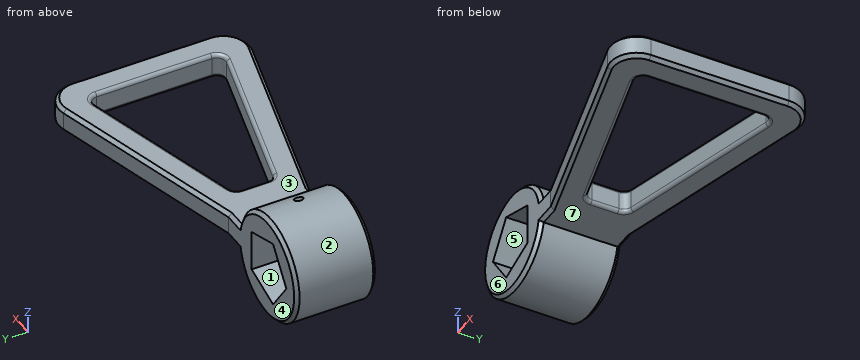
```python
from build123d import *

# Parameters (mm, degrees)
BOSS_EXTRUDE2_DEPTH     = 7
SKETCH2_R               = 30
BOSS_EXTRUDE4_DEPTH     = 23
CUT_EXTRUDE1_DEPTH      = 46
CUT_EXTRUDE2_REACH      = 185.241
CUT_EXTRUDE2_END_RADIUS = 30
SKETCH4_R               = 2.5
FILLET1_R               = 5
CHAMFER1_SIZE           = 2
FILLET2_R               = 2


with BuildPart() as part:
    # Sketch1 → Boss-Extrude2 (new, symmetric)
    with BuildSketch(Plane.XY):
        with BuildLine():
            Line((174, -39.356811193), (174, 39.356811193))
            ThreePointArc((174, 39.356811193), (168.131421435, 51.257111298), (155.117714323, 53.845698587))
            Line((155.117714323, 53.845698587), (40, 23))
            Line((40, 23), (30, 23))
            Line((30, 23), (0, 23))
            Line((0, 23), (0, -23))
            Line((0, -23), (30, -23))
            Line((30, -23), (40, -23))
            Line((40, -23), (155.117714323, -53.845698587))
            ThreePointArc((155.117714323, -53.845698587), (168.131421435, -51.257111298), (174, -39.356811193))
        make_face()
        Polygon((159, -39.356811193), (159, 39.356811193), (55, 11.49009518), (55, -11.49009518), align=None, mode=Mode.SUBTRACT)
    extrude(amount=BOSS_EXTRUDE2_DEPTH, both=True)

    # Sketch2 → Boss-Extrude4 (add, symmetric)
    with BuildSketch(Plane(origin=(0, 0, 0), x_dir=(1, 0, 0), z_dir=(0, 1, 0))):
        Circle(SKETCH2_R)
    extrude(amount=BOSS_EXTRUDE4_DEPTH, both=True)

    # Sketch3 → Cut-Extrude1 (cut)
    with BuildSketch(Plane(origin=(0, 23, 0), x_dir=(1, 0, 0), z_dir=(0, 1, 0))):
        Polygon((16.099689438, 11.697109064), (-6.149534157, 18.926320036), (-19.900310562, 0), (-6.149534157, -18.926320036), (16.099689438, -11.697109064), align=None)
    extrude(amount=-CUT_EXTRUDE1_DEPTH, mode=Mode.SUBTRACT)

    # Cut-Extrude2: up to this cylinder (the profile starts inside it)
    cut_extrude2_end = Plane(origin=(0, 0, 0), z_dir=(0, -1, 0)) * Cylinder(CUT_EXTRUDE2_END_RADIUS, 431.482, mode=Mode.PRIVATE)
    # Sketch4 → Cut-Extrude2 (cut, up to the surface)
    with BuildSketch(Plane(origin=(4.975077641, 0, 15.31171455), x_dir=(-0.9510565162951536, 0, 0.30901699437494745), z_dir=(-0.3090169943749474, 0, -0.9510565162951535)), mode=Mode.PRIVATE) as cut_extrude2_sk1:
        Circle(SKETCH4_R)
    cut_extrude2_tool1 = extrude(cut_extrude2_sk1.sketch, amount=-CUT_EXTRUDE2_REACH, mode=Mode.PRIVATE) & cut_extrude2_end
    add(cut_extrude2_tool1.solids().sort_by_distance((4.975078, 0, 15.311715))[0], mode=Mode.SUBTRACT)

    # Fillet1
    fillet1_edges = [part.edges().sort_by_distance(p)[0] for p in [
        (55, -11.49009518, 0),
        (159, -39.356811193, 0),
        (159, 39.356811193, 0),
        (55, 11.49009518, 0),
    ]]
    fillet(fillet1_edges, radius=FILLET1_R)

    # Chamfer1
    chamfer1_edges = [part.edges().sort_by_distance(p)[0] for p in [
        (34.585952146, 23, 7),
        (97.558857162, -38.422849294, -7),
        (34.585952146, 23, -7),
        (97.558857162, 38.422849294, -7),
        (168.131421435, 51.257111298, -7),
        (97.558857162, -38.422849294, 7),
        (168.131421435, -51.257111298, 7),
        (174, 0, 7),
        (168.131421435, 51.257111298, 7),
        (34.585952146, -23, -7),
        (34.585952146, -23, 7),
        (-30, -23, 0),
        (-30, 23, 0),
        (97.558857162, 38.422849294, 7),
        (174, 0, -7),
        (168.131421435, -51.257111298, -7),
    ]]
    chamfer(chamfer1_edges, length=CHAMFER1_SIZE)

    # Fillet2
    fillet2_edges = [part.edges().sort_by_distance(p)[0] for p in [
        (105.705904774, -25.076701416, -7),
        (105.705904774, -25.076701416, 7),
        (159, 0, -7),
        (159, 0, 7),
        (105.705904774, 25.076701416, -7),
        (105.705904774, 25.076701416, 7),
        (55, 0, -7),
        (55, 0, 7),
        (157.043807145, -36.80745103, -7),
        (157.043807145, -36.80745103, 7),
        (157.043807145, 36.80745103, -7),
        (157.043807145, 36.80745103, 7),
        (56.033233299, -10.697267385, -7),
        (56.033233299, -10.697267385, 7),
        (56.033233299, 10.697267385, -7),
        (56.033233299, 10.697267385, 7),
    ]]
    fillet(fillet2_edges, radius=FILLET2_R)


solid = part.part
```
The listing builds one solid part. Answer for the finished solid, in the listing's coordinates (mm). Face numbers are marked on the shaded views. A direction names the side the tool comes from. Coordinates: 2 decimals unless noted, no trailing zeros. Write each loop counter-clockwise with the first axis right and the second up, starting at its lowest first coordinate (ties: lowest second). Pieces come first, ordered by that corner, then holes. Notation, with made-up numbers: (-10, 13.25) - (48, 13.25) arc R18 cw to (48, 48.25) - close; hole circle Ø2 at (-4, 45). An arc over 180 degrees is marked (long way). Return JSON: item names as keys, results as strings. Group by question number.
Q1. Flat-ended cylindrical pins translate along their axes: pin 1 Ø12 at (y, z) = (-32, 22.5) entering from -X; pin 2 Ø3 at (y, z) = (-9.5, -2) entering from -X; pin 3 Ø10 at (x, z) = (42, -7.5) entering from -Y; pin 4 Ø12 at (x, z) = (11, 22.5) entering from -Y. Find the tip coordinate at first contact, or state that the pin passes through.
Q2. The part is cut by section B-B on x = 32. Write down the section's boundary in (y, z).
Q3. Which of the six approach directions +Z, -Z, +X, -X, +Y, -Y give full straight-line access (tool end or side, diameter ignored) to the marked faces 4, 5, 6 and 7?
Q4. The part is cut by section A-A on x = 0. Write down the section's boundary in (y, z), and give its area (3 significant figures).
Q5. The part is cut by section C-C on y = -10.5. State how many separate pieces and enclosed holes the cut face has, and give its area (3 significant figures).
Q6. For a pull along X with two mould halves and no side action, classify the marked faces 1, 2 and 3 as +X half, -X half, draft (parallel to the pull), parting line (faces both ways), or undercut.
Q7. Find the intervals of material crossed by line 1 along Y through (x, z) = (66, 2.5); line 2 along X through (y, z) = (-12, 4.5); line 3 along Y through (x, z) = (66.5, 1), in increasing order. Write a range as [from, to].
Evaluation:
{
 "1": {"pin 1": "passes through", "pin 2": "stops at x = -30", "pin 3": "stops at y = -24.7", "pin 4": "stops at y = -23"},
 "2": {"outline": "(-23, -5) - (-21, -7) - (21, -7) - (23, -5) - (23, 5) - (21, 7) - (-21, 7) - (-23, 5) - close"},
 "3": {"face 4": "+Z, -Z, -X, +Y", "face 5": "+Y, -Y", "face 6": "+Z, -Z, -X, -Y", "face 7": "-Z, +X, +Y, -Y"},
 "4": {"outline": "(-23, -28) - (-21, -30) - (21, -30) - (23, -28) - (23, -16.93) - (-23, -16.93) - close; (-23, 16.93) - (23, 16.93) - (23, 28) - (21, 30) - (-21, 30) - (-23, 28) - close", "area": "1,190 mm2"},
 "5": {"separate pieces": "2", "enclosed holes": "1", "area": "2,450 mm2"},
 "6": {"face 1": "undercut", "face 2": "parting line", "face 3": "draft"},
 "7": {"line 1": "y = [-29.97, -14.44], [14.44, 29.97]", "line 2": "x = [-29.66, -16.63], [16.1, 57.53], [159, 174]", "line 3": "y = [-30.1, -14.57], [14.57, 30.1]"}
}
